```python
from build123d import *

# Parameters (mm, degrees)
SKETCH1_W              = 125
SKETCH1_H              = 43
BOSS_EXTRUDE1_DEPTH    = 55
CUT_EXTRUDE1_START     = -43
CUT_EXTRUDE1_OUTLINE_W = 6
CUT_EXTRUDE1_OUTLINE_H = 18
CUT_EXTRUDE1_OUTLINE_R = 7.5
CUT_EXTRUDE1_DEPTH     = 43
SKETCH8_R              = 160
CUT_EXTRUDE3_DEPTH     = 133.846716181
SKETCH3_W              = 13.5
SKETCH3_H              = 31.460130223
SKETCH3_H_2            = 5.539869777
SKETCH3_H_3            = 6.548888359
CUT_EXTRUDE2_DEPTH     = 139.247061452


# Read off the part's stored shape, not the designer's step: Cut-Extrude1
with BuildPart() as part:
    # Sketch1 → Boss-Extrude1 (new body)
    with BuildSketch(Plane(origin=(0, 0, 0), x_dir=(1, 0, 0), z_dir=(0, 1, 0))):
        Rectangle(SKETCH1_W, SKETCH1_H)
    extrude(amount=BOSS_EXTRUDE1_DEPTH)

    # Cut-Extrude1 outline → Cut-Extrude1 (cut)
    with BuildSketch(Plane.XY.offset(21.5).offset(CUT_EXTRUDE1_START)):
        with Locations((-59.5, 9)):
            Rectangle(CUT_EXTRUDE1_OUTLINE_W, CUT_EXTRUDE1_OUTLINE_H)
        with Locations((59.5, 9)):
            Rectangle(CUT_EXTRUDE1_OUTLINE_W, CUT_EXTRUDE1_OUTLINE_H)
        with BuildLine():
            Line((-62.5, 55), (-62.5, 25.142135624))
            ThreePointArc((-62.5, 25.142135624), (-62.119397663, 27.055552786), (-61.035533906, 28.67766953))
            Line((-61.035533906, 28.67766953), (-39.106601718, 50.606601718))
            ThreePointArc((-39.106601718, 50.606601718), (-34.240251487, 53.858192988), (-28.500000002, 55))
            Line((-28.500000002, 55), (-62.5, 55))
        make_face()
        with BuildLine():
            ThreePointArc((58.994623203, 28.311253379), (61.529461255, 26.500180908), (62.5, 23.539869777))
            Line((62.5, 23.539869777), (62.5, 55))
            Line((62.5, 55), (-28.500000002, 55))
            ThreePointArc((-28.500000002, 55), (-26.231990093, 54.82754636), (-24.016130392, 54.314150807))
            Line((-24.016130392, 54.314150807), (58.994623203, 28.311253379))
        make_face()
        with Locations((-28.5, 40)):
            Circle(CUT_EXTRUDE1_OUTLINE_R)
    extrude(amount=CUT_EXTRUDE1_DEPTH, mode=Mode.SUBTRACT)

    # Sketch8 → Cut-Extrude3 (cut, through all)
    with BuildSketch(Plane(origin=(56.5, 0, 0), x_dir=(0, 0, -1), z_dir=(1, 0, 0))):
        with Locations((0, -158.548888359)):
            Circle(SKETCH8_R)
    extrude(amount=-CUT_EXTRUDE3_DEPTH, mode=Mode.SUBTRACT)

    # Sketch3 → Cut-Extrude2 (cut, through all)
    with BuildSketch(Plane(origin=(62.5, 0, 0), x_dir=(0, 0, -1), z_dir=(1, 0, 0))):
        with Locations((-6.75, 39.269934889)):
            Rectangle(SKETCH3_W, SKETCH3_H)
        with Locations((6.75, 39.269934889)):
            Rectangle(SKETCH3_W, SKETCH3_H)
        with Locations((6.75, 20.769934888)):
            Rectangle(SKETCH3_W, SKETCH3_H_2)
        with Locations((-6.75, 20.769934888)):
            Rectangle(SKETCH3_W, SKETCH3_H_2)
        with Locations((-6.75, 14.725555821)):
            Rectangle(SKETCH3_W, SKETCH3_H_3)
        with Locations((6.75, 14.725555821)):
            Rectangle(SKETCH3_W, SKETCH3_H_3)
    extrude(amount=-CUT_EXTRUDE2_DEPTH, mode=Mode.SUBTRACT)


solid = part.part
```
Model file for the job. Use its own axes, mm. A direction names the side the tool comes from. Round coordinates to 2 decimals unless told otherwise and drop trailing zeros. Write each loop counter-clockwise with the first axis right and the second up, starting at its lowest first coordinate (ties: lowest second). Pieces come first, ordered by that corner, then holes. Notation, with made-up numbers: M 86.5,57 L 126.5,57 A22 ccw 126.5,86 Z; hole C 79,64 d4. An arc over 180 degrees is marked long. Put each result on its own line as item: value.
Item 1: Mould opens along Y. For faces 4 (the cylindrical face through (-30.13, 32.68, 17.44)), 5 (the flat face through (62.5, 21, 18)), 6 (the cylindrical face through (61.5, 26.54, 17.44)), 7 (the flat face through (59, 18, -18)) say: +Y half, -Y half, draft (parallel to the pull), parting line (faces both ways), or undercut.
Responses:
face 4: undercut
face 5: draft
face 6: +Y half
face 7: -Y half
Item 2: Cut at D-D (y = 8). List the corners of the cut face in (x, z).
Responses:
outline: M -56.5,-21.5 L 56.5,-21.5 L 56.5,21.5 L -56.5,21.5 Z
Item 3: Probe L1, parallel to Z at x = -36, y = 30; L2, parallel to Y at x = -28, z = -16; L3, parallel to Y at x = -28, z = 15. List the from-to ranges inside material, lowest first. Write a range as from..to.
Responses:
L1: -21.5..-13.5, 13.5..21.5
L2: 0.65..32.52, 47.48..54.99
L3: 0.75..32.52, 47.48..54.99
Item 4: Tool access for faces 1 (the flat face through (56.5, 9, 0)), 2 (the cylindrical face through (0.79, 1.45, -0.3)), 3 (the flat face through (-56.5, 9, 0)): list every direction of +Z, -Z, +X, -X, +Y, -Y with a clear straight run to the whole face (end or side of a thin tool).
Responses:
face 1: +Z, -Z, +X, -Y
face 2: +X, -X, -Y
face 3: +Z, -Z, -X, -Y
Item 5: Cut at B-B (x = -3). List the corners of the cut face in (y, z).
Responses:
outline: M 0,-21.5 L 47.73,-21.5 L 47.73,-13.5 L 11.45,-13.5 L 11.45,13.5 L 47.73,13.5 L 47.73,21.5 L 0,21.5 A160 cw Z
Item 6: Cut at C-C (z = -18). List the corners of the cut face in (x, y).
Responses:
outline: M -62.5,18 L -56.5,18 L -56.5,0.44 L 56.5,0.44 L 56.5,18 L 62.5,18 L 62.5,23.54 A5 ccw 58.99,28.31 L -24.02,54.31 A15 ccw -39.11,50.61 L -61.04,28.68 A5 ccw -62.5,25.14 Z; hole C -28.5,40 d15
Item 7: Cut at A-A (y = 40). List the corners of the cut face in (x, z).
Responses:
outline: M -49.71,-21.5 L -36,-21.5 L -36,-13.5 L -49.71,-13.5 Z; M -49.71,13.5 L -36,13.5 L -36,21.5 L -49.71,21.5 Z; M -21,-21.5 L 21.68,-21.5 L 21.68,-13.5 L -21,-13.5 Z; M -21,13.5 L 21.68,13.5 L 21.68,21.5 L -21,21.5 Z
Item 8: Flat gauge pins, fed straight in: P1, Ø13.5, axis at x = -28.5, y = 40, coming from the -Z side; P2, Ø20, axis at y = 5, z = 2, coming from the +X side; P3, Ø8, axis at x = -23.5, z = -6.5, coming from the +Y side; P4, Ø6.5, axis at x = 58.5, z = -16.5, coming from the -Y side. Where does each tip first touch, or does it go through?
Responses:
P1: through
P2: x = 56.5
P3: y = 11.45
P4: y = 0.31
